Check sheet for the modelled part. Datum: model origin and axes. Units: mm. Round coordinates to 2 decimals unless told otherwise and drop trailing zeros. Write each loop counter-clockwise with the first axis right and the second up, starting at its lowest first coordinate (ties: lowest second). Pieces come first, ordered by that corner, then holes. Notation, with made-up numbers: (40, 34) - (64, 34) arc R13 cw to (64, 54) - close; hole circle Ø1 at (87, 70). An arc over 180 degrees is marked (long way). Answer as a JSON object with one key per item and string values. Group by question number.
Item 1: Sectioned sample at A-A on y = 0. Record the boundary of the cut face in (x, z), plus the area to 3 significant figures.
Item 2: Thickness scan on line 1 (Y direction, x = 0, z = 27.5); line 2 (X direction, y = -14, z = 30.5); line 3 (X direction, y = 7.5, z = 37). Record the ranges inside material, lowest first.
Item 3: Sectioned sample at C-C on z = 28.5. Record the boundary of the cut face in (x, y).
Item 4: Release check for a two-part mould opening along X. For faces 1 (the cylindrical face through (27.45, 8.65, 19.72)), 2 (the flat face through (-38.1, 0, 20)), 3 (the flat face through (0, 38.1, 20)) record: pulls with the +X half, pulls with the -X half, needs draft (parallel to the pull), parting line crosses it, or undercut.
```python
from build123d import *

# Parameters (mm, degrees)
F0_R      = 28.781011
F1_DEPTH  = 40
F1_FACE_R = 28.781011
F2_DEPTH  = 10
F3_DEPTH  = 20


with BuildPart() as f1:
    # F0 (on Top) → F1 (new body)
    with BuildSketch(Plane.XY):
        with BuildLine():
            Line((30.48, 38.1), (-30.48, 38.1))
            ThreePointArc((-30.48, 38.1), (-35.868154, 35.868154), (-38.1, 30.48))
            Line((-38.1, 30.48), (-38.1, -30.48))
            ThreePointArc((-38.1, -30.48), (-35.868154, -35.868154), (-30.48, -38.1))
            Line((-30.48, -38.1), (30.48, -38.1))
            ThreePointArc((30.48, -38.1), (35.868154, -35.868154), (38.1, -30.48))
            Line((38.1, -30.48), (38.1, 30.48))
            ThreePointArc((38.1, 30.48), (35.868154, 35.868154), (30.48, 38.1))
        make_face()
        Circle(F0_R, mode=Mode.SUBTRACT)
    extrude(amount=F1_DEPTH)

    # F1_face (on face) → F2 (join)
    with BuildSketch(Plane(origin=(0, 0, 0), x_dir=(1, 0, 0), z_dir=(0, 0, -1))):
        with BuildLine():
            Line((-30.48, -38.1), (30.48, -38.1))
            ThreePointArc((30.48, -38.1), (35.868154, -35.868154), (38.1, -30.48))
            Line((38.1, -30.48), (38.1, 30.48))
            ThreePointArc((38.1, 30.48), (35.868154, 35.868154), (30.48, 38.1))
            Line((30.48, 38.1), (-30.48, 38.1))
            ThreePointArc((-30.48, 38.1), (-35.868154, 35.868154), (-38.1, 30.48))
            Line((-38.1, 30.48), (-38.1, -30.48))
            ThreePointArc((-38.1, -30.48), (-35.868154, -35.868154), (-30.48, -38.1))
        make_face()
        Circle(F1_FACE_R, mode=Mode.SUBTRACT)
    extrude(amount=-F2_DEPTH)

    # F0 (on Top) → F3 (join)
    with BuildSketch(Plane.XY):
        with BuildLine():
            Line((30.48, 38.1), (-30.48, 38.1))
            ThreePointArc((-30.48, 38.1), (-35.868154, 35.868154), (-38.1, 30.48))
            Line((-38.1, 30.48), (-38.1, -30.48))
            ThreePointArc((-38.1, -30.48), (-35.868154, -35.868154), (-30.48, -38.1))
            Line((-30.48, -38.1), (30.48, -38.1))
            ThreePointArc((30.48, -38.1), (35.868154, -35.868154), (38.1, -30.48))
            Line((38.1, -30.48), (38.1, 30.48))
            ThreePointArc((38.1, 30.48), (35.868154, 35.868154), (30.48, 38.1))
        make_face()
        Circle(F0_R, mode=Mode.SUBTRACT)
    extrude(amount=F3_DEPTH)


solid = f1.part
```
Completed:
{
 "1": {"outline": "(-38.1, 0) - (-28.78, 0) - (-28.78, 40) - (-38.1, 40) - close; (28.78, 0) - (38.1, 0) - (38.1, 40) - (28.78, 40) - close", "area": "746 mm²"},
 "2": {"line 1": "-38.1 to -28.78, 28.78 to 38.1", "line 2": "-38.1 to -25.15, 25.15 to 38.1", "line 3": "-38.1 to -27.79, 27.79 to 38.1"},
 "3": {"outline": "(-38.1, -30.48) arc R7.62 ccw to (-30.48, -38.1) - (30.48, -38.1) arc R7.62 ccw to (38.1, -30.48) - (38.1, 30.48) arc R7.62 ccw to (30.48, 38.1) - (-30.48, 38.1) arc R7.62 ccw to (-38.1, 30.48) - close; hole circle Ø57.56 at (0, 0)"},
 "4": {"face 1": "undercut", "face 2": "pulls with the -X half", "face 3": "needs draft"}
}
